from build123d import *

# Parameters (mm, degrees)
F0_W      = 270
F0_H      = 250
F4_REACH  = 517.9673898595
F5_W      = 263
F5_H      = 236
F6_DEPTH  = 36
F8_DEPTH  = 250.001
F10_D     = 3.5
F10_DEPTH = 12
F10_TIP   = 1.0515060833


with BuildPart() as f4:
    f4_end = Plane(origin=(25.6515107494, 0, -145.4769465589), x_dir=(0.984807753, 0, 0.1736481777), z_dir=(-0.1736481777, 0, 0.984807753))
    # F0 (on Top) → F4 (new body, up to a plane its end follows)
    with BuildSketch(Plane.XY):
        with Locations((135, 125)):
            Rectangle(F0_W, F0_H)
    f4_long = extrude(amount=-F4_REACH, mode=Mode.PRIVATE)
    add(split(f4_long, bisect_by=f4_end, keep=Keep.TOP, mode=Mode.PRIVATE))

    # F5 (on face) → F6 (cut)
    with BuildSketch(Plane.XY):
        with Locations((138.5, 125)):
            Rectangle(F5_W, F5_H)
    extrude(amount=-F6_DEPTH, mode=Mode.SUBTRACT)

    # F7 (on face) → F8 (cut, through all)
    with BuildSketch(Plane.XZ):
        with BuildLine():
            Line((270, -46.2953201601), (221.9611568908, -54.7658643223))
            ThreePointArc((221.9611568908, -54.7658643223), (207.7658643223, -75.0388431092), (228.0388431092, -89.2341356777))
            Line((228.0388431092, -89.2341356777), (270, -81.8352515761))
            Line((270, -81.8352515761), (270, -46.2953201601))
        make_face()
    extrude(amount=-F8_DEPTH, mode=Mode.SUBTRACT)

    # F10
    with Locations(Plane.XY):
        with Locations((3.5, 64.25), (3.5, 125), (3.5, 185.75), (3.5, 246.5), (3.5, 3.5), (65.75, 3.5), (135, 3.5), (204.25, 3.5), (266.5, 3.5), (266.500000929, 246.5237677097), (204.25, 246.5237677097), (135, 246.5237677097), (65.75, 246.5)):
            Hole(F10_D / 2, depth=F10_DEPTH)
            with Locations((0, 0, -(F10_DEPTH + F10_TIP / 2))):  # 118° drill point
                Cone(0, F10_D / 2, F10_TIP, mode=Mode.SUBTRACT)


solid = f4.part
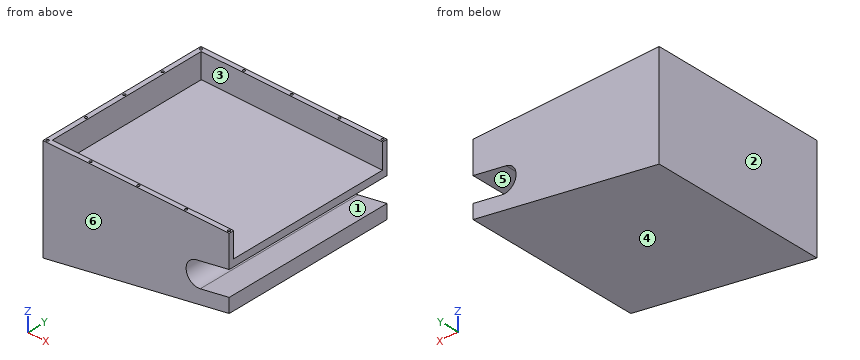
Here's how the part is built. I have some questions about the finished solid (model axes, mm). Face numbers are marked on the shaded views. A direction names the side the tool comes from. Coordinates: 2 decimals unless noted, no trailing zeros. Loops run counter-clockwise (first coordinate to the right, second up) from the corner with the lowest first, then second, coordinate; pieces in that order, holes last.
1. For the marked faces 1, 2 and 3, which set-ups out of +Z, -Z, +X, -X, +Y, -Y let a thin tool reach every point of the face, with its end or its side?
2. Imagine slicing it at D-D, the plane z = -72. Please give me the cut outline in (x, y), and give its area (3 significant figures).
3. Imagine slicing it at C-C, the plane x = 117.5. Please give me the cut outline in (y, z).
4. If we mould it in two halves opening along Z, with no side actions, what happens to the marked faces 4, 5 and 6? For each: pulls with the +Z half, pulls with the -Z half, needs draft (parallel to the pull), parting line crosses it, or undercut.
5. I need wall thicknesses on L1, parallel to Y at x = 204, z = -3; L2, parallel to Y at x = 3.5, z = -4; L3, parallel to Y at x = 65.75, z = -6.5. Which ranges of each line are inside material? Lowest first, please.
6. Imagine slicing it at B-B, the plane x = 215. Please give me the cut outline in (y, z), and give its area (3 significant figures).
7. Imagine slicing it at A-A, the plane y = 50.5. Please give me the cut outline in (x, z).
8. For P1, Ø3, axis at x = 135, y = 246.52, coming from the +Z side; P2, Ø3, axis at x = 115, y = 72.5, coming from the -Z side; P3, Ø4, axis at x = 230, y = 38, coming from the +Z side, each with a flat end and sliding along its axis, tell me the tip position at first contact or that it passes through.
Taken from the geometry:
1. face 1: +Y, -Y
1. face 2: +Z, -Z, -X, +Y, -Y
1. face 3: +Z, +X
2. outline: (0, 0) - (207.5, 0) - (207.5, 250) - (0, 250) - close
2. area: 51,900 mm2
3. outline: (0, -129.28) - (250, -129.28) - (250, 0) - (243, 0) - (243, -36) - (7, -36) - (7, 0) - (0, 0) - close
4. face 4: pulls with the -Z half
4. face 5: undercut
4. face 6: needs draft
5. L1: y = 0 to 1.77, 5.23 to 7, 243 to 244.79, 248.26 to 250
5. L2: y = 0 to 1.75, 5.25 to 62.5, 66 to 123.25, 126.75 to 184, 187.5 to 244.75, 248.25 to 250
5. L3: y = 0 to 1.75, 5.25 to 7, 243 to 244.75, 248.25 to 250
6. outline: (0, -112.09) - (250, -112.09) - (250, -86.36) - (0, -86.36) - close; (0, -57.64) - (250, -57.64) - (250, 0) - (243, 0) - (243, -36) - (7, -36) - (7, 0) - (0, 0) - close
6. area: 12,300 mm2
7. outline: (0, -150) - (270, -102.39) - (270, -81.84) - (228.04, -89.23) arc R17.5 cw to (221.96, -54.77) - (270, -46.3) - (270, -36) - (7, -36) - (7, 0) - (0, 0) - close
8. P1: stops at z = -12.15
8. P2: stops at z = -129.99
8. P3: stops at z = -36
